CAD build for the part. Positions are in the model's coordinates, mm. A direction names the side the tool comes from. Round coordinates to 2 decimals unless told otherwise and drop trailing zeros. Order: outer loops, then holes, each group sorted by start corner. A loop starts at its lowest first (then second) coordinate and runs counter-clockwise, first axis right, second up. Notation, with made-up numbers: (4.5, 79.5) - (18.5, 79.5) arc R20 cw to (18.5, 86.5) - close; hole circle Ø7 at (15.25, -35). An arc over 180 degrees is marked (long way). Use one line per item in the form item = value. Start each with the question number.
Autodesk Inventor part; units mm, degrees
ref_plane "Начальная плоскость" through (0, 0, 10) normal (0, 0, 1) x (1, 0, 0)
ref_plane "Конечная плоскость" through (0, 0, 280) normal (0, 0, 1) x (1, 0, 0)
ref_plane "РабПлоскость4" through (300, -4.7971, 280) normal (0, 0, 1) x (1, 0, 0)
ref_plane "Начальная плоскость" through (0, 0, 10) normal (0, 0, 1) x (1, 0, 0)
ref_plane "Конечная плоскость" through (0, 0, 280) normal (0, 0, 1) x (1, 0, 0)
sketch "Эскиз" plane through (0, 0, 0) normal (0, 0, 1) x (1, 0, 0)
  line L0 (-14.4349, 0) -> (14.4349, 0)
  line L1 (0, -14) -> (0, 14)
  line L2 (0, 0) -> (7.5, 7.5) construction
  circle A0 centre (7.5, 7.5) radius 1.65 construction
  line L3 (5.85, 9.15) -> (9.15, 9.15)
  line L4 (9.15, 9.15) -> (9.15, 5.85)
  line L5 (9.15, 5.85) -> (5.85, 5.85)
  line L6 (5.85, 5.85) -> (5.85, 9.15)
  line L7 (3.235, 8.1636) -> (4.72, 9.9636)
  line L8 (4.7971, 10) -> (8.5, 10)
  line L9 (3.3121, 8) -> (4.95, 8)
  line L10 (4.95, 8) -> (4.95, 5.7985)
  line L11 (4.95, 5.7985) -> (2.6515, 3.5)
  line L12 (0, 3.5) -> (2.6515, 3.5)
  circle A1 centre (0, 0) radius 2.5
  line L13 (8.1636, 3.235) -> (9.9636, 4.72)
  line L14 (10, 4.7971) -> (10, 8.5)
  line L15 (8, 3.3121) -> (8, 4.95)
  line L16 (8, 4.95) -> (5.7985, 4.95)
  line L17 (5.7985, 4.95) -> (3.5, 2.6515)
  line L18 (3.5, 0) -> (3.5, 2.6515)
  arc A2 (10, 8.5) -> (8.5, 10) centre (8.5, 8.5) ccw
  line L19 (0, 0) -> (-7.5, 7.5) construction
  circle A3 centre (-7.5, 7.5) radius 1.65 construction
  line L20 (-5.85, 9.15) -> (-9.15, 9.15)
  line L21 (-9.15, 9.15) -> (-9.15, 5.85)
  line L22 (-9.15, 5.85) -> (-5.85, 5.85)
  line L23 (-5.85, 5.85) -> (-5.85, 9.15)
  line L24 (-3.235, 8.1636) -> (-4.72, 9.9636)
  line L25 (-4.7971, 10) -> (-8.5, 10)
  line L26 (-3.3121, 8) -> (-4.95, 8)
  line L27 (-4.95, 8) -> (-4.95, 5.7985)
  line L28 (-4.95, 5.7985) -> (-2.6515, 3.5)
  line L29 (0, 3.5) -> (-2.6515, 3.5)
  line L30 (-3.5, 0) -> (-3.5, 2.6515)
  line L31 (-5.7985, 4.95) -> (-3.5, 2.6515)
  line L32 (-8, 4.95) -> (-5.7985, 4.95)
  line L33 (-8, 3.3121) -> (-8, 4.95)
  line L34 (-8.1636, 3.235) -> (-9.9636, 4.72)
  line L35 (-10, 4.7971) -> (-10, 8.5)
  arc A4 (-8.5, 10) -> (-10, 8.5) centre (-8.5, 8.5) ccw
  line L36 (0, 14) -> (0, -14)
  line L37 (0, 0) -> (7.5, -7.5) construction
  circle A5 centre (7.5, -7.5) radius 1.65 construction
  line L38 (5.85, -9.15) -> (9.15, -9.15)
  line L39 (9.15, -9.15) -> (9.15, -5.85)
  line L40 (9.15, -5.85) -> (5.85, -5.85)
  line L41 (5.85, -5.85) -> (5.85, -9.15)
  line L42 (3.235, -8.1636) -> (4.72, -9.9636)
  line L43 (4.7971, -10) -> (8.5, -10)
  line L44 (3.3121, -8) -> (4.95, -8)
  line L45 (4.95, -8) -> (4.95, -5.7985)
  line L46 (4.95, -5.7985) -> (2.6515, -3.5)
  line L47 (0, -3.5) -> (2.6515, -3.5)
  line L48 (3.5, 0) -> (3.5, -2.6515)
  line L49 (5.7985, -4.95) -> (3.5, -2.6515)
  line L50 (8, -4.95) -> (5.7985, -4.95)
  line L51 (8, -3.3121) -> (8, -4.95)
  line L52 (8.1636, -3.235) -> (9.9636, -4.72)
  line L53 (10, -4.7971) -> (10, -8.5)
  arc A6 (8.5, -10) -> (10, -8.5) centre (8.5, -8.5) ccw
  line L54 (0, 0) -> (-7.5, -7.5) construction
  line L55 (-4.95, -8) -> (-4.95, -5.7985)
  line L56 (-3.3121, -8) -> (-4.95, -8)
  line L57 (-5.7985, -4.95) -> (-3.5, -2.6515)
  line L58 (-4.95, -5.7985) -> (-2.6515, -3.5)
  line L59 (-3.5, 0) -> (-3.5, -2.6515)
  line L60 (0, -3.5) -> (-2.6515, -3.5)
  circle A7 centre (-7.5, -7.5) radius 1.65 construction
  line L61 (-5.85, -5.85) -> (-5.85, -9.15)
  line L62 (-5.85, -9.15) -> (-9.15, -9.15)
  line L63 (-9.15, -9.15) -> (-9.15, -5.85)
  line L64 (-9.15, -5.85) -> (-5.85, -5.85)
  line L65 (-3.235, -8.1636) -> (-4.72, -9.9636)
  line L66 (-8, -4.95) -> (-5.7985, -4.95)
  line L67 (-8, -3.3121) -> (-8, -4.95)
  line L68 (-8.1636, -3.235) -> (-9.9636, -4.72)
  line L69 (-4.7971, -10) -> (-8.5, -10)
  line L70 (-10, -4.7971) -> (-10, -8.5)
  arc A8 (-10, -8.5) -> (-8.5, -10) centre (-8.5, -8.5) ccw
  arc A9 (3.235, 8.1636) -> (3.3121, 8) centre (3.3121, 8.1) ccw
  arc A10 (4.7971, 10) -> (4.72, 9.9636) centre (4.7971, 9.9) ccw
  arc A11 (8, 3.3121) -> (8.1636, 3.235) centre (8.1, 3.3121) ccw
  arc A12 (9.9636, 4.72) -> (10, 4.7971) centre (9.9, 4.7971) ccw
  arc A13 (-3.3121, 8) -> (-3.235, 8.1636) centre (-3.3121, 8.1) ccw
  arc A14 (-4.72, 9.9636) -> (-4.7971, 10) centre (-4.7971, 9.9) ccw
  arc A15 (-8.1636, 3.235) -> (-8, 3.3121) centre (-8.1, 3.3121) ccw
  arc A16 (-10, 4.7971) -> (-9.9636, 4.72) centre (-9.9, 4.7971) ccw
  arc A17 (-8, -3.3121) -> (-8.1636, -3.235) centre (-8.1, -3.3121) ccw
  arc A18 (-9.9636, -4.72) -> (-10, -4.7971) centre (-9.9, -4.7971) ccw
  arc A19 (-3.235, -8.1636) -> (-3.3121, -8) centre (-3.3121, -8.1) ccw
  arc A20 (-4.7971, -10) -> (-4.72, -9.9636) centre (-4.7971, -9.9) ccw
  arc A21 (4.72, -9.9636) -> (4.7971, -10) centre (4.7971, -9.9) ccw
  arc A22 (3.3121, -8) -> (3.235, -8.1636) centre (3.3121, -8.1) ccw
  arc A23 (8.1636, -3.235) -> (8, -3.3121) centre (8.1, -3.3121) ccw
  arc A24 (10, -4.7971) -> (9.9636, -4.72) centre (9.9, -4.7971) ccw
  point P0 (3.1, 8)
  point P1 (4.75, 10)
  point P2 (7.5, 9.15)
  point P3 (8, 3.1)
  point P4 (10, 4.75)
  point P5 (7.5, 5.85)
  point P6 (9.15, 7.5)
  point P7 (-3.1, 8)
  point P8 (-4.75, 10)
  point P9 (-7.5, 9.15)
  point P10 (-8, 3.1)
  point P11 (-10, 4.75)
  point P12 (-7.5, 5.85)
  point P13 (-9.15, 7.5)
  point P14 (3.1, -8)
  point P15 (4.75, -10)
  point P16 (7.5, -9.15)
  point P17 (8, -3.1)
  point P18 (10, -4.75)
  point P19 (7.5, -5.85)
  point P20 (9.15, -7.5)
  point P21 (-3.1, -8)
  point P22 (-7.5, -5.85)
  point P23 (-7.5, -9.15)
  point P24 (-9.15, -7.5)
  point P25 (-4.75, -10)
  point P26 (-8, -3.1)
  point P27 (-10, -4.75)
  dimension "d0" = 45
  dimension "d1" = 3.3
  dimension "d2" = 1.5
  dimension "d3" = 1.2
  dimension "d4" = 5
  dimension "d5" = 6.5
  dimension "d6" = 15
  dimension "d7" = 20
  dimension "d8" = 9.9
  dimension "d9" = 9.5
  dimension "d10" = 6.2
  dimension "d11" = 2
  dimension "d18" = 0.1
  dimension "d19" = 0.1
extrude "Тело" add sketch "Эскиз" along normal up to surface (270 mm away) from surface at 10 contours A1 L1 L12 L11 L10 L9 A9 L7 A10 L8 A2 L14 A12 L13 A11 L15 L16 L17 L18 L0 | L0 L48 L49 L50 L51 A23 L52 A24 L53 A6 L43 A21 L42 A22 L44 L45 L46 L47 L1 A1 | A1 L0 L30 L31 L32 L33 A15 L34 A16 L35 A4 L25 A14 L24 A13 L26 L27 L28 L29 L1 | L1 L60 L58 L55 L56 A19 L65 A20 L69 A8 L70 A18 L68 A17 L67 L66 L57 L59 L0 A1
sketch "Эскиз2" plane through (0, 0, 0) normal (0, 0, 1) x (1, 0, 0)
  line L0 (0, 0) -> (10, 0)
ref_plane "РабПлоскость3" through (0, 0, 0) normal (0, -1, 0) x (1, 0, 0)
sketch "Эскиз3" plane through (0, 0, 0) normal (0, -1, 0) x (1, 0, 0)
  line L0 (-2, 10) -> (12, 10)
  line L1 (-2, 280) -> (12, 280)
  dimension "d25" = 270
ref_plane "РабПлоскость4" through (300, -4.7971, 280) normal (0, 0, 1) x (1, 0, 0)
split "Разделение1" plane through (300, -4.7971, 280) removes the side toward (0, 0, 1)
ref_plane "РабПлоскость5" through (300, -8.5, 10) normal (0, 0, -1) x (-1, 0, 0)
split "Разделение2" plane through (300, -8.5, 10) removes the side toward (0, 0, -1)
properties part number "короткая палка"
(1) Slice it at C-C (z = 181.5). Give the number of separate pieces and of enclosed holes in the cut face, and give its area (3 significant figures).
(2) Which spindle directions (+Z, -Z, +X, -X, +Y, -Y) get a long thin tool onto all of the face, cutting with end or side? Do faces 1 (the flat face through (0, 3.5, 143)), 2 (the flat face through (3.5, 0, 143)), 3 (the flat face through (0, -3.5, 143)), 4 (the flat face through (-3.5, 0, 143)). Say none if no direction does.
(3) Flat gauge pins, fed straight in: P1, Ø0.5, axis at x = 4, z = 189, coming from the +Y side; P2, Ø2.5, axis at x = 0, z = 81, coming from the -Y side; P3, Ø0.8, axis at x = -4, z = 180, coming from the -Y side. Where does each tip first touch, or does it go through?
(4) Slice it at A-A (y = 0). Give the cut face in (x, z).
(5) Wall check: line 1 (Y direction, x = -7, z = 265); line 2 (Y direction, x = 8.5, z = 246); line 3 (Y direction, x = 0, z = 83). Give the ranges that are in metal, low to high. Write a range as [from, to].
Results list:
q1.separate_pieces = 1
q1.enclosed_holes = 5
q1.area = 115 mm²
q2.face_1 = +Z, -Z, +Y
q2.face_2 = +Z, -Z, +X
q2.face_3 = +Z, -Z, -Y
q2.face_4 = +Z, -Z, -X
q3.P1 = 9.39
q3.P2 = -3.5
q3.P3 = -9.58
q4.outline = (-3.5, 10) - (-2.5, 10) - (-2.5, 280) - (-3.5, 280) - close; (2.5, 10) - (3.5, 10) - (3.5, 280) - (2.5, 280) - close
q5.line_1 = [-10, -9.15], [-5.85, -4.95], [4.95, 5.85], [9.15, 10]
q5.line_2 = [-10, -9.15], [-5.85, -3.51], [3.51, 5.85], [9.15, 10]
q5.line_3 = [-3.5, -2.5], [2.5, 3.5]
